Verification items for the finished model (mm, model axes). Face numbers are marked on the shaded views. Give positions to 0.01 mm unless a question says otherwise; leave off trailing zeros. Loops run counter-clockwise (first coordinate to the right, second up) from the corner with the lowest first, then second, coordinate; pieces in that order, holes last. Notation, with made-up numbers: M 54,-28 L 71,-28 A23 cw 71,-7 Z; hole C 13.5,53.25 d9. An arc over 180 degrees is marked long. Answer in a Markdown table with one row per item.
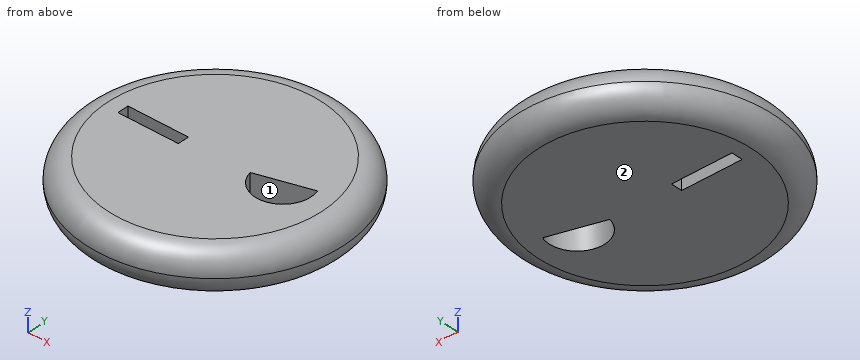
```python
from build123d import *

# Parameters (mm, degrees)
F0_R     = 76.327515992
F0_W     = 35.994451493
F0_H     = 6.7489598878
F1_DEPTH = 25.4
F2_R     = 12.69999


# Not quite as in the source:
# - a fillet or chamfer is up to 0.001 mm smaller than in the source, because OpenCascade refuses the exact size


with BuildPart() as f1:
    # F0 (on Top) → F1 (new body)
    with BuildSketch(Plane.XY):
        Circle(F0_R)
        with BuildLine():
            ThreePointArc((0, 71.7222208521), (50.7152687262, 50.7152687262), (71.7222208521, 0))
            ThreePointArc((71.7222208521, 0), (50.7152687263, -50.7152687262), (0, -71.7222208521))
            ThreePointArc((0, -71.7222208521), (-71.7222208521, 0), (0, 71.7222208521))
        make_face(mode=Mode.SUBTRACT)
        with BuildLine():
            ThreePointArc((0, -71.7222208521), (50.7152687263, -50.7152687262), (71.7222208521, 0))
            ThreePointArc((71.7222208521, 0), (50.7152687262, 50.7152687262), (0, 71.7222208521))
            Line((0, 71.7222208521), (0, -71.7222208521))
        make_face()
        with BuildLine():
            ThreePointArc((51.5885779704, 10.5423588198), (40.6190136024, -10.9400752111), (19.8122242535, 1.2625405457))
            Line((19.8122242535, 1.2625405457), (51.5885779704, 10.5423588198))
        make_face(mode=Mode.SUBTRACT)
        with BuildLine():
            Line((0, -71.7222208521), (0, 71.7222208521))
            ThreePointArc((0, 71.7222208521), (-71.7222208521, 0), (0, -71.7222208521))
        make_face()
        with Locations((-36.8380714208, 0)):
            Rectangle(F0_W, F0_H, mode=Mode.SUBTRACT)
    extrude(amount=F1_DEPTH)

    # F2 (radius 12.7 in the source; OpenCascade refuses exactly that, so slightly less here)
    f2_edges = [f1.edges().sort_by_distance(p)[0] for p in [
        (-76.327516, 0, 25.4),
        (-76.327516, 0, 0),
    ]]
    fillet(f2_edges, radius=F2_R)


solid = f1.part
```
Item 1: Scan lines: L1, parallel to X at y = -2.5, z = 23.25; L2, parallel to Y at x = -19, z = 4.75; L3, parallel to Y at x = 24, z = 2.5. Record each from-to range of solid material in increasing order. Write a range as [from, to].
Reported:
| item | result |
|---|---|
| L1 | x = [-70.65, -54.84], [-18.84, 21.17], [50.77, 70.65] |
| L2 | y = [-71.03, -3.37], [3.37, 71.03] |
| L3 | y = [-67.03, -6.5], [2.49, 67.03] |
Item 2: Go/stop test with flat-tipped pins: pin 1 (3.5 mm diameter, centred on y = 1, z = 12.5, fed in from +X); pin 2 (1 mm diameter, centred on y = 38.5, z = 10, fed in from +X); pin 3 (12 mm diameter, centred on x = 43.5, z = 6.5, fed in from +Y); pin 4 (10 mm diameter, centred on y = -35.5, z = 20.5, fed in from +X). Record where each tip stops, or that it passes through.
Reported:
| item | result |
|---|---|
| pin 1 | stops at x = 76.33 |
| pin 2 | stops at x = 65.89 |
| pin 3 | stops at y = 65.55 |
| pin 4 | stops at x = 68.51 |
Item 3: Release check for a two-part mould opening along X. For the marked faces 1 and 2 record: released by +X, released by -X, zero draft, split by the parting line, or undercut.
Reported:
| item | result |
|---|---|
| face 1 | undercut |
| face 2 | zero draft |
Item 4: Sectioned sample at A-A (z = 10). Record the cut outline in (x, y), and give its area (3 significant figures).
Reported:
| item | result |
|---|---|
| outline | C 0,0 d152.07; hole M -54.84,-3.37 L -18.84,-3.37 L -18.84,3.37 L -54.84,3.37 Z; hole M 19.81,1.26 A16.58 ccw long 51.59,10.54 Z |
| area | 17,500 mm^2 |
